Source: CAD feature listing. Evaluate the final solid. Frame: model axes, mm. Face numbers are marked on the shaded views. A direction names the side the tool comes from. Coordinates: 2 decimals unless noted, no trailing zeros. Order: outer loops, then holes, each group sorted by start corner. A loop starts at its lowest first (then second) coordinate and runs counter-clockwise, first axis right, second up. Notation, with made-up numbers: (13.25, 6) - (23.25, 6) arc R13 ccw to (23.25, 20) - close; hole circle Ø2 at (7, -5). An arc over 180 degrees is marked (long way). One line per question, with ' | ' between items. Start each with the question number.
(1) Line query: line 1 along X through (y, z) = (5.75, 29.5); line 2 along Z through (x, y) = (38.1, -1.2); line 3 along Y through (x, z) = (5, 23.5). Output: solid intervals per line, ascending.
(2) Access query for the marked faces 5, 6 and 7. Directions: +Z, -Z, +X, -X, +Y, -Y. A direction counts if a zero-diameter tool reaches every point of the face in a straight line with its end or side. Return the directions, or none.
(3) Section B-B (z = 35). Return the cut outline in (x, y).
(4) Section A-A (x = 38.1). Return the cut outline in (y, z), then the cut area to 3 significant figures.
(5) Section C-C (y = 2). Return the cut outline in (x, z), then the cut area to 3 significant figures.
(6) Draft query along X for the marked faces 1, 2, 3 and 4. Return one class per face: +X half, -X half, draft (parallel to the pull), parting line (faces both ways), or undercut.
(7) Section D-D (x = 2). Return the cut outline in (y, z).
(8) Contact query for flat-ended pins moving along their axis: P1, Ø4, axis at y = 4.5, z = 23, coming from the +X side; P2, Ø4, axis at x = -39, z = 28.5, coming from the +Y side; P3, Ø10, axis at x = -7, z = 23.5, coming from the -Y side. Output: stop coordinate, or through.
from build123d import *

# Parameters (mm, degrees)
BOSS_EXTRUDE1_DEPTH   = 39.878
F_4_CLEARANCE_HOLE1_D = 2.9464
FILLET1_R             = 2.54
FILLET2_R             = 2.54


with BuildPart() as part:
    # Sketch1 → Boss-Extrude1 (new body)
    with BuildSketch(Plane.XY):
        Polygon((-43.02125, 0), (-30.32125, 0), (-30.32125, 12.7), (30.32125, 12.7), (30.32125, 0), (43.02125, 0), (43.02125, -2.38125), (27.94, -2.38125), (27.94, 10.31875), (-27.94, 10.31875), (-27.94, -2.38125), (-43.02125, -2.38125), align=None)
    extrude(amount=BOSS_EXTRUDE1_DEPTH)

    # #4 Clearance Hole1 (through all)
    with Locations(Plane(origin=(0, 0, 0), x_dir=(1, 0, 0), z_dir=(0, 1, 0))):
        with Locations((-38.1, -20.948579073)):
            f_4_clearance_hole1 = Hole(F_4_CLEARANCE_HOLE1_D / 2)

    # Mirror1: #4 Clearance Hole1 across plane
    add(f_4_clearance_hole1.mirror(Plane(origin=(0, 0, 0), x_dir=(0, 0, 1), z_dir=(1, 0, 0))), mode=Mode.SUBTRACT)

    # Fillet1
    # the kernel refuses this fillet: 2.54 mm, written as the material it takes off along each edge
    with BuildSketch(Plane(origin=(-27.94, 10.31875, 39.878), x_dir=(-1, 0, 0), z_dir=(0, -1, 0))) as fillet1_piece_1:
        with BuildLine():
            CenterArc((FILLET1_R, FILLET1_R), FILLET1_R, 180, 90)
            Line((0, FILLET1_R), (0, 0))
            Line((0, 0), (FILLET1_R, 0))
        make_face()
    extrude(amount=19.05, mode=Mode.SUBTRACT)

    # Fillet2
    # the kernel refuses this fillet: 2.54 mm, written as the material it takes off along each edge
    with BuildSketch(Plane(origin=(27.94, 10.31875, 39.878), x_dir=(0, 0, -1), z_dir=(-1, 0, 0))) as fillet2_piece_1_section:
        with BuildLine():
            CenterArc((2.535034208, -2.54), FILLET2_R, 90, 86.416678302)
            Line((0, -2.38125), (0, 0))
            Line((0, 0), (2.535034208, 0))
        make_face()
    fillet2_piece_1 = extrude(amount=64.598835521, mode=Mode.PRIVATE)
    fillet2_piece_1 = fillet2_piece_1 - Plane(origin=(-30.48, 11.003720119, 37.338), x_dir=(-1, 0, 0), z_dir=(0, 1, 0)) * Cylinder(2.54, 140, mode=Mode.PRIVATE)
    add(fillet2_piece_1, mode=Mode.SUBTRACT)


solid = part.part
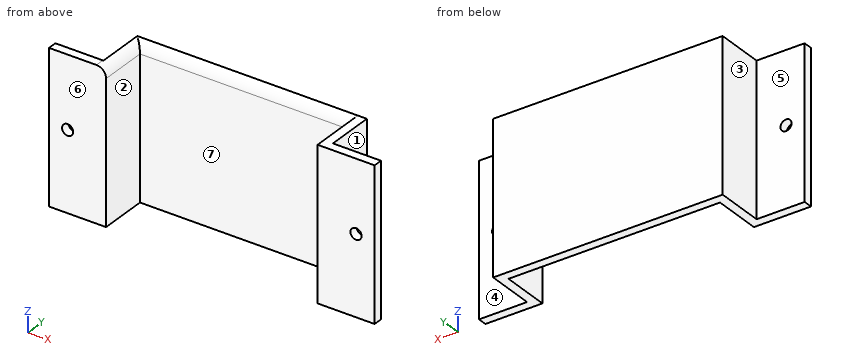
Response values:
1) line 1: x = -30.32 to -27.94, 27.94 to 30.32 | line 2: z = 0 to 19.48, 22.42 to 39.88 | line 3: y = 10.32 to 12.7
2) face 5: +Z, -Z, -X, +Y | face 6: +Z, -Z, +X, -X, -Y | face 7: +Z, -Z, -Y
3) outline: (-43.02, -2.38) - (-27.94, -2.38) - (-27.94, 10.32) - (27.94, 10.32) - (27.94, -2.38) - (43.02, -2.38) - (43.02, 0) - (30.32, 0) - (30.32, 12.7) - (-30.32, 12.7) - (-30.32, 0) - (-43.02, 0) - close
4) outline: (-2.38, 0) - (0, 0) - (0, 19.48) - (-2.38, 19.48) - close; (-2.38, 22.42) - (0, 22.42) - (0, 39.88) - (-2.38, 39.88) - close | area: 87.9 mm²
5) outline: (-30.32, 0) - (-27.94, 0) - (-27.94, 37.34) arc R2.54 ccw to (-30.32, 39.87) - close; (27.94, 0) - (30.32, 0) - (30.32, 39.88) - (27.94, 39.88) - close | area: 189 mm²
6) face 1: +X half | face 2: undercut | face 3: -X half | face 4: draft
7) outline: (10.32, 0) - (12.7, 0) - (12.7, 39.88) arc R2.54 ccw to (10.32, 37.34) - close
8) P1: stops at x = 30.32 | P2: stops at y = 0 | P3: stops at y = 10.32
